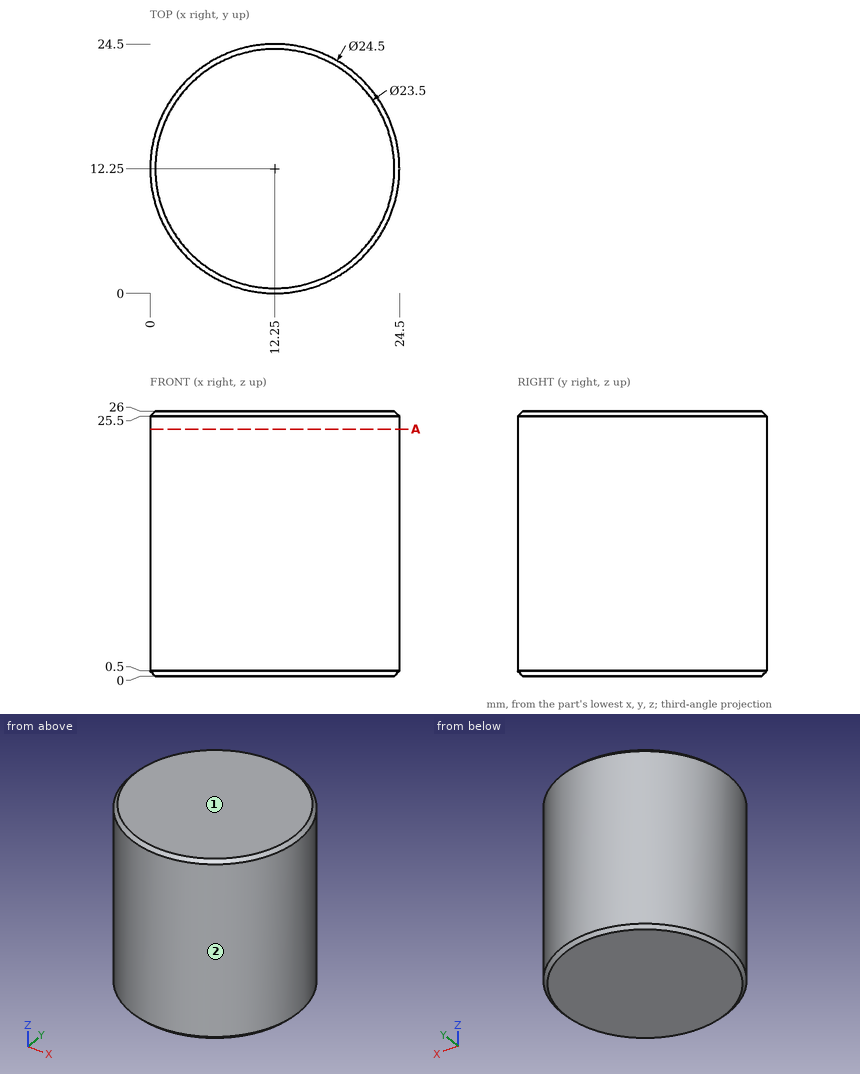
Print and shaded views of the part. All mm, measured from the part's lowest x, y and z. Give positions to 0.01 mm unless a question says otherwise; leave off trailing zeros. Write each loop counter-clockwise with the first axis right and the second up, starting at its lowest first coordinate (ties: lowest second). Pieces come first, ordered by that corner, then holes. Notation, with made-up numbers: (-38, 9) - (9, 9) arc R24 ccw to (9, 41) - close; hole circle Ø3 at (30.5, -10.75). An arc over 180 degrees is marked (long way). Put each result on its own line as item: value.
(1) Drop flat-ended pins along their axis: pin 1 Ø12 at (y, z) = (7.5, 5.5) entering from -X; pin 2 Ø10 at (y, z) = (3, 4.5) entering from -X; pin 3 Ø1 at (x, z) = (11.5, 21) entering from -Y; pin 4 Ø3 at (x, z) = (16.5, 11) entering from -Y. Give the stop position or say it passes through.
Working result:
pin 1: x = 0
pin 2: x = 0.76
pin 3: y = 0
pin 4: y = 0.31
(2) Pull direction X, two halves, no side cores. Call the marked faces 1 and 2: released by +X, released by -X, zero draft, split by the parting line, or undercut.
Working result:
face 1: zero draft
face 2: split by the parting line
(3) Saw through at A-A (z = 24.25). List the corners of the cut face in (x, y).
Working result:
outline: circle Ø24.5 at (12.25, 12.25)
(4) Wall check: L1, parallel to Y at x = 12.5, z = 9.25; L2, parallel to X at y = 6, z = 10.25; L3, parallel to X at y = 8.5, z = 17.25. Give the ranges that are in metal, low to high.
Working result:
L1: 0 to 24.5
L2: 1.71 to 22.79
L3: 0.59 to 23.91
